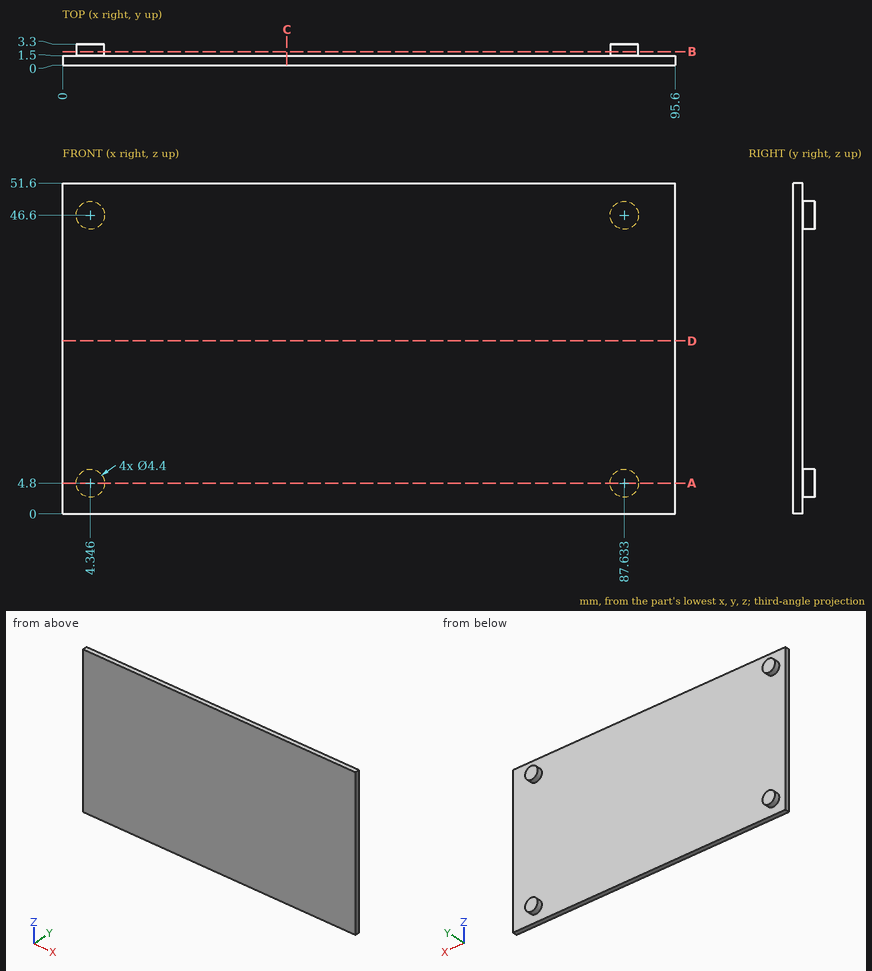
Can you work these out from the drawing? Everything is in mm from the part's minimum corner. Round coordinates to 2 decimals unless told otherwise and drop trailing zeros. Order: outer loops, then holes, each group sorted by start corner. A loop starts at its lowest first (then second) coordinate and runs counter-clockwise, first axis right, second up.
(1) If we section it at B-B (y = 2.1): Please give me the cut outline in (x, z), plus the area to 3 significant figures.
Results are:
outline: circle Ø4.4 at (4.35, 4.8); circle Ø4.4 at (4.35, 46.6); circle Ø4.4 at (87.63, 4.8); circle Ø4.4 at (87.63, 46.6)
area: 60.8 mm2
(2) If we section it at C-C (x = 35): Please give me the cut outline in (y, z), plus the area to 3 significant figures.
Results are:
outline: (0, 0) - (1.5, 0) - (1.5, 51.6) - (0, 51.6) - close
area: 77.4 mm2
(3) If I drill on L1, parallel to Y at x = 23.5, z = 38.5; L2, parallel to X at y = 2.4, z = 4.5 (1 decimal); L3, parallel to Z at x = 86, y = 2.9 (1 decimal), over which ranges is the centre line in solid material (lowest first)?
Results are:
L1: y = 0 to 1.5
L2: x = 2.2 to 6.5, 85.5 to 89.8
L3: z = 3.3 to 6.3, 45.1 to 48.1
(4) I'm going to push flat-ended pins straight in: pin 1 (1.5 mm diameter, centred on x = 27.5, z = 8.5, fed in from -Y); pin 2 (15.5 mm diameter, centred on x = 39, z = 25, fed in from +Y). Where does each tip first touch, or does it pass through?
Results are:
pin 1: stops at y = 0
pin 2: stops at y = 1.5
(5) If we section it at A-A (z = 4.8): Please give me the cut outline in (x, y), plus the area to 3 significant figures.
Results are:
outline: (0, 0) - (95.6, 0) - (95.6, 1.5) - (89.83, 1.5) - (89.83, 3.3) - (85.43, 3.3) - (85.43, 1.5) - (6.55, 1.5) - (6.55, 3.3) - (2.15, 3.3) - (2.15, 1.5) - (0, 1.5) - close
area: 159 mm2
(6) If we section it at D-D (z = 27): Please give me the cut outline in (x, y).
Results are:
outline: (0, 0) - (95.6, 0) - (95.6, 1.5) - (0, 1.5) - close
